```python
from build123d import *

# Parameters (mm, degrees)
F0_R     = 11.15
F1_DEPTH = 7
F2_W     = 41.241116
F2_H     = 1.306281
F3_DEPTH = 2


with BuildPart() as f1:
    # F0 (on Top) → F1 (new body)
    with BuildSketch(Plane.XY):
        Polygon((14.433757, 25), (-14.433757, 25), (-28.867513, 0), (-14.433757, -25), (14.433757, -25), (28.867513, 0), align=None)
        Circle(F0_R, mode=Mode.SUBTRACT)
    extrude(amount=F1_DEPTH)

    # F2 (on face) → F3 (cut)
    with BuildSketch(Plane.XY.offset(7)):
        with Locations((13.249409, -18.661137)):
            Rectangle(F2_W, F2_H)
        Polygon((-1.3396, 38.33625), (19.280958, 2.620396), (20.41223, 3.273536), (-0.208328, 38.989391), align=None)
        Polygon((-32.530367, -20.328253), (-11.909808, 15.387601), (-13.041081, 16.040742), (-33.661639, -19.675113), align=None)
    extrude(amount=-F3_DEPTH, mode=Mode.SUBTRACT)


solid = f1.part
```
CAD build for the part. Positions are in the model's coordinates, mm. A direction names the side the tool comes from. Round coordinates to 2 decimals unless told otherwise and drop trailing zeros. Write each loop counter-clockwise with the first axis right and the second up, starting at its lowest first coordinate (ties: lowest second). Pieces come first, ordered by that corner, then holes. Notation, with made-up numbers: (-28.75, -38.75) - (0.25, -38.75) arc R21 ccw to (0.25, 0.25) - close; hole circle Ø11 at (32.5, 84.25). An arc over 180 degrees is marked (long way). Return JSON: item names as keys, results as strings. Group by question number.
Item 1: Band-saw the part on C-C on x = 17. List the corners of the cut face in (y, z), plus the area to 3 significant figures.
Item 2: Band-saw the part on B-B on z = 4.25. List the corners of the cut face in (x, y), plus the area to 3 significant figures.
Item 3: Band-saw the part on A-A on x = 0. List the corners of the cut face in (y, z), plus the area to 3 significant figures.
Item 4: Band-saw the part on D-D on y = -16. List the corners of the cut face in (x, z), plus the area to 3 significant figures.
Item 5: Probe probe 1 along Y at (x, z) = (2, 6.75); probe 2 along X at (y, z) = (14.5, 5.5); probe 3 along Y at (x, z) = (-0.5, 2.5). List the from-to ranges inside material, lowest first.
Item 6: 3-axis set-ups, long thin cutter, end or side, ignore diameter. For faces 4 (the face through (-19.225, 5.33, 6.014)), 5 (the face through (-0.4, 11.5, 0)), 6 (the face through (5, -19.314, 6)): which of +Z, -Z, +X, -X, +Y, -Y reach the whole face in a straight line?
Item 7: Mould opens along Y. For faces 1 (the face through (21.752, 12.325, 3.451)), 2 (the face through (21.55, -12.675, 3.451)), 3 (the face through (5, -18.008, 6)) say: +Y half, -Y half, draft (parallel to the pull), parting line (faces both ways), or undercut.
Item 8: Flat gauge pins, fed straight in: pin 1 Ø1.5 at (y, z) = (-14, 2) entering from -X; pin 2 Ø0.6 at (x, z) = (6.5, 6.5) entering from +Y; pin 3 Ø1.4 at (y, z) = (-18.5, 6) entering from +X; pin 4 Ø2 at (y, z) = (4.5, 3) entering from +X. Where does each tip first touch, or does it go through?
Resolved:
{
 "1": {"outline": "(-20.56, 0) - (20.56, 0) - (20.56, 7) - (9.18, 7) - (9.18, 5) - (6.57, 5) - (6.57, 7) - (-18.01, 7) - (-18.01, 5) - (-19.31, 5) - (-19.31, 7) - (-20.56, 7) - close", "area": "280 mm²"},
 "2": {"outline": "(-28.87, 0) - (-14.43, -25) - (14.43, -25) - (28.87, 0) - (14.43, 25) - (-14.43, 25) - close; hole circle Ø22.3 at (0, 0)", "area": "1,770 mm²"},
 "3": {"outline": "(-25, 0) - (-11.15, 0) - (-11.15, 7) - (-18.01, 7) - (-18.01, 5) - (-19.31, 5) - (-19.31, 7) - (-25, 7) - close; (11.15, 0) - (25, 0) - (25, 7) - (11.15, 7) - close", "area": "191 mm²"},
 "4": {"outline": "(-19.63, 0) - (19.63, 0) - (19.63, 7) - (-19.63, 7) - close", "area": "275 mm²"},
 "5": {"probe 1": "y = -25 to -19.31, -18.01 to -10.97, 10.97 to 25", "probe 2": "x = -20.5 to -13.93, -12.42 to 12.42, 13.93 to 20.5", "probe 3": "y = -25 to -11.14, 11.14 to 25"},
 "6": {"face 4": "+Z", "face 5": "-Z, +X, -X, +Y, -Y", "face 6": "+Z, +X"},
 "7": {"face 1": "+Y half", "face 2": "-Y half", "face 3": "undercut"},
 "8": {"pin 1": "stops at x = -21.22", "pin 2": "stops at y = 25", "pin 3": "stops at x = 18.59", "pin 4": "stops at x = 26.85"}
}
